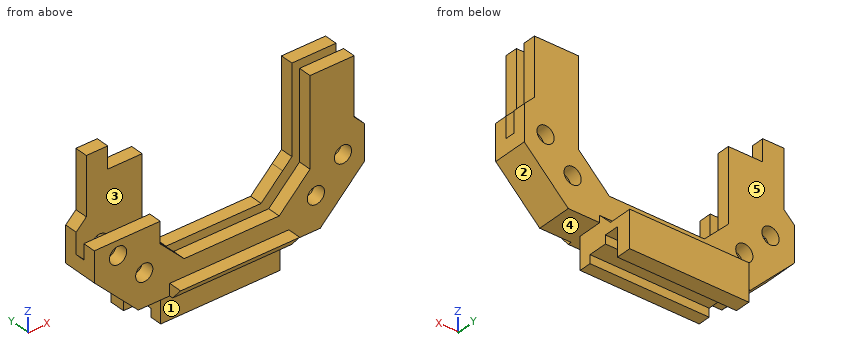
Autodesk Inventor part; units mm, degrees
ref_plane "Work Plane1" through (59.9208, 47.0911, 21.911) normal (0, 1, 0) x (-1, 0, 0)
ref_plane "Work Plane2" through (59.9208, 45.8611, 21.911) normal (0, -1, 0) x (1, 0, 0)
ref_plane "Work Plane13" through (59.9208, 43.8611, -18.7491) normal (1, 0, 0) x (0, 0, -1)
ref_plane "Work Plane1" through (59.9208, 47.0911, 21.911) normal (0, 1, 0) x (-1, 0, 0)
sketch "Sketch1" plane through (59.9208, 47.0911, 21.911) normal (0, 1, 0) x (-1, 0, 0)
  circle A0 centre (-16.808, -43.6345) radius 1.27
  circle A1 centre (12.5729, -47.6345) radius 1.27
  circle A2 centre (16.4459, -43.6345) radius 1.27
  circle A3 centre (-12.808, -47.6345) radius 1.27
  line L0 (10.208, -33.8805) -> (10.208, -44.6601)
  line L1 (10.208, -44.6601) -> (6.6725, -48.1956)
  circle A4 centre (-16.808, -43.6345) radius 1.27
  circle A5 centre (12.5729, -47.6345) radius 1.27
  circle A6 centre (16.4459, -43.6345) radius 1.27
  circle A7 centre (-12.8081, -47.6345) radius 1.27
  line L2 (19.708, -15.6655) -> (-19.708, -15.6655)
  line L3 (0, -15.6655) -> (0, -20.8781)
  line L4 (6.6725, -48.1956) -> (-7.3796, -48.1956)
  line L5 (-19.958, -43.8381) -> (-12.8316, -50.9645)
  line L6 (-12.8316, -50.9645) -> (12.8316, -50.9645)
  line L7 (-19.958, -40.6601) -> (-19.958, -43.8381)
  line L8 (0, -48.1956) -> (0, -46.7038)
  line L9 (19.958, -43.8381) -> (12.8316, -50.9645)
  line L10 (19.958, -40.6601) -> (19.958, -43.8381)
  line L11 (-11.938, -30.6601) -> (-11.938, -43.6372)
  line L12 (-10.5616, -45.0137) -> (-11.938, -43.6372)
  line L13 (-10.5616, -45.0137) -> (-7.3796, -48.1956)
  line L14 (15.2967, -30.6601) -> (18.458, -30.6601)
  line L15 (18.458, -30.6601) -> (18.458, -39.1601)
  line L16 (-18.458, -39.1601) -> (-18.458, -30.6601)
  line L17 (-18.458, -30.6601) -> (-11.938, -30.6601)
  line L18 (10.208, -33.8805) -> (15.2967, -33.8805)
  line L19 (15.2967, -33.8805) -> (15.2967, -30.6601)
  line L20 (-19.958, -40.6601) -> (-18.458, -39.1601)
  line L21 (19.958, -40.6601) -> (18.458, -39.1601)
  point P0 (-19.708, -43.6601)
  point P1 (-6.6725, -48.1956)
  dimension "d14" = 5
  dimension "d15" = 135
  dimension "d18" = 2.54
extrude "Extrusion1" add sketch "Sketch1" along normal blind 2
ref_plane "Work Plane2" through (59.9208, 45.8611, 21.911) normal (0, -1, 0) x (1, 0, 0)
sketch "Sketch2" plane through (59.9208, 45.8611, 21.911) normal (0, -1, 0) x (1, 0, 0)
  line L0 (-10.208, -33.8805) -> (-10.208, -44.6601)
  line L1 (-10.208, -44.6601) -> (-6.6725, -48.1956)
  line L2 (-6.6725, -48.1956) -> (7.3796, -48.1956)
  circle A0 centre (16.808, -43.6345) radius 1.27
  circle A1 centre (-12.5729, -47.6345) radius 1.27
  circle A2 centre (-16.4459, -43.6345) radius 1.27
  circle A3 centre (12.808, -47.6345) radius 1.27
  line L3 (19.958, -40.6601) -> (19.958, -43.8381)
  line L4 (19.958, -43.8381) -> (12.8316, -50.9645)
  line L5 (12.8316, -50.9645) -> (-12.8316, -50.9645)
  line L6 (-12.8316, -50.9645) -> (-19.958, -43.8381)
  line L7 (-19.958, -43.8381) -> (-19.958, -40.6601)
  line L8 (7.3796, -48.1956) -> (11.938, -43.6372)
  line L9 (11.938, -43.6372) -> (11.938, -30.6601)
  line L10 (11.938, -30.6601) -> (18.458, -30.6601)
  line L11 (18.458, -30.6601) -> (18.458, -39.1601)
  line L12 (-18.458, -39.1601) -> (-18.458, -30.6601)
  line L13 (-18.458, -30.6601) -> (-15.2967, -30.6601)
  line L14 (-15.2967, -30.6601) -> (-15.2967, -33.8805)
  line L15 (-15.2967, -33.8805) -> (-10.208, -33.8805)
  line L16 (18.458, -39.1601) -> (19.958, -40.6601)
  line L17 (-19.958, -40.6601) -> (-18.458, -39.1601)
  circle A4 centre (-16.4459, -43.6345) radius 1.27
  line L18 (-19.958, -43.8381) -> (-19.958, -40.6601)
  line L19 (-19.958, -41.5123) -> (-10.208, -41.5123)
  line L20 (-10.208, -33.8805) -> (-10.208, -44.6601)
  point P0 (-59.9208, -21.911)
extrude "Extrusion2" add sketch "Sketch2" along normal blind 2 contours L0 L1 L2 L8 L9 L10 L11 L16 L3 L4 L5 L6 L7 L19
sketch "Sketch4" plane through (79.8789, 45.8611, -18.7491) normal (1, 0, 0) x (0, 0, -1)
  line L0 (0, 1.23) -> (3.178, 1.23)
  line L1 (0, 0) -> (-1.5, 0)
  line L2 (0, 1.23) -> (0, 0)
  line L3 (-12.1065, -0.085) -> (12.1065, -0.085)
  line L4 (12.1065, -0.085) -> (12.1065, 1.315)
  line L5 (12.1065, 1.315) -> (-12.1065, 1.315)
  line L6 (-12.1065, 1.315) -> (-12.1065, -0.085)
  line L7 (-12.1065, -0.085) -> (12.1065, 1.315) construction
  line L8 (12.1065, -0.085) -> (-12.1065, 1.315) construction
  point P0 (0, 0.615)
  dimension "d73" = 1.4
extrude "Extrusion3" cut sketch "Sketch4" against normal through all
sketch "Sketch5" plane through (59.9208, 43.8611, 21.911) normal (0, -1, 0) x (1, 0, 0)
  line L0 (-19.708, -43.6601) -> (-19.708, -40.6601)
  line L1 (-12.6424, -50.7145) -> (-19.708, -43.6601)
  line L2 (12.728, -50.7145) -> (-12.6424, -50.7145)
  line L3 (19.708, -43.7345) -> (12.728, -50.7145)
  line L4 (-13.4529, -52.4645) -> (13.4529, -52.4645)
  line L5 (19.708, -43.7345) -> (19.708, -40.6601)
  line L6 (-12.8316, -50.9145) -> (12.8316, -50.9145)
  line L7 (12.8316, -50.9645) -> (11.3316, -52.4645)
  line L8 (-19.958, -43.8381) -> (-12.8316, -50.9645)
  line L9 (-12.8316, -50.9645) -> (-11.3316, -52.4645)
  line L10 (-12.8316, -50.9645) -> (-10.7103, -50.9645) construction
  line L11 (12.8316, -50.9145) -> (12.8816, -50.9145)
  line L12 (-12.8316, -50.9645) -> (12.8316, -50.9645)
  line L13 (12.8316, -50.9645) -> (12.8816, -50.9145)
  line L14 (12.8316, -50.9645) -> (19.958, -43.8381)
  line L15 (-12.8316, -50.9145) -> (-12.8816, -50.9145)
  line L16 (-12.8316, -50.9645) -> (-12.8816, -50.9145)
  line L17 (12.8109, -50.9145) -> (19.958, -43.7673)
  line L18 (-19.958, -43.7673) -> (-12.8109, -50.9145)
  line L19 (-19.958, -45.9594) -> (-13.4529, -52.4645)
  line L20 (13.4529, -52.4645) -> (19.958, -45.9594)
  line L21 (-19.958, -43.7673) -> (-19.958, -45.9594)
  line L22 (12.8316, -50.9645) -> (19.958, -43.8381)
  line L23 (19.958, -43.8381) -> (19.958, -45.9594)
  line L24 (19.958, -43.8381) -> (19.958, -43.7673)
  line L25 (19.958, -43.8381) -> (19.958, -40.6601)
  dimension "d29" = 0.2
  dimension "d62" = 45
  dimension "d74" = 0.05
  dimension "d75" = 0.05
  dimension "d76" = 1.5
  dimension "d77" = 1.5
extrude "Extrusion4" add sketch "Sketch5" against normal up to surface (5.23 mm away)
ref_plane "Work Plane13" through (59.9208, 43.8611, -18.7491) normal (1, 0, 0) x (0, 0, -1)
ref_plane "Work Plane14" through (53.2483, 46.4761, -26.2847) normal (0, 1, 0) x (1, 0, 0)
sketch "Sketch18" plane through (59.9208, 43.8611, -18.7491) normal (1, 0, 0) x (0, 0, -1)
  line L0 (12.8044, 1.651) -> (16.5534, 1.651)
  line L1 (16.5534, 1.651) -> (16.5534, 3.4515)
  line L2 (16.5534, 3.4515) -> (15.3033, 3.4515)
  line L3 (15.3033, 3.4515) -> (15.3033, 6.2794)
  line L4 (15.3033, 6.2794) -> (14.0544, 6.2794)
  line L5 (14.0544, 6.2794) -> (14.0544, 8.48)
  line L6 (14.0544, 8.48) -> (18.2804, 8.48)
  line L7 (18.2804, 8.48) -> (18.2804, 10.73)
  line L8 (18.2804, 10.73) -> (12.8044, 10.73)
  line L9 (12.8044, 7.23) -> (12.8044, 10.73)
  line L10 (11.8044, 0) -> (11.8044, 5.23)
  line L11 (11.8044, 5.23) -> (11.8044, 0)
  line L12 (11.8044, 5.23) -> (10.8044, 5.23)
  line L13 (12.8044, 1.651) -> (11.8044, 1.651)
  line L14 (12.8044, 7.23) -> (10.8044, 5.23)
  line L15 (11.8044, 0) -> (10.0544, 0)
  line L16 (10.0544, 0) -> (10.0544, -2)
  line L17 (10.0544, -2) -> (11.8044, -0.5316)
  line L18 (11.8044, -0.5316) -> (11.8044, 0)
  point P0 (12.8044, 5.23)
  point P1 (11.8044, 1.651)
  dimension "d182" = 2
  dimension "d183" = 2
  dimension "d184" = 1.75
  dimension "d185" = 2
  dimension "d186" = 50
extrude "Extrusion12" add sketch "Sketch18" along normal blind 8.804 and the other way blind 8.804
ref_plane "Work Plane19" through (51.1168, 52.1911, -37.0296) normal (0, -1, 0) x (1, 0, 0)
ref_plane "Work Plane20" through (68.7248, 50.1406, -34.2524) normal (0, 0, -1) x (-1, 0, 0)
properties part number "Button Holder"
Here's how the part is built. I have some questions about the finished solid (model axes, mm). Face numbers are marked on the shaded views. A direction names the side the tool comes from. Give positions to 0.01 mm unless a question says otherwise; leave off trailing zeros. Order: outer loops, then holes, each group sorted by start corner. A loop starts at its lowest first (then second) coordinate and runs counter-clockwise, first axis right, second up. Notation, with made-up numbers: (55, 74.5) - (69, 74.5) arc R15 cw to (69, 96.5) - close; hole circle Ø11 at (80.25, 52). An arc over 180 degrees is marked (long way). Answer as a JSON object with one key per item and string values. Group by question number.
Item 1: If we mould it in two halves opening along Y, with no side actions, what happens to the marked faces 3, 4 and 5? For each: pulls with the +Y half, pulls with the -Y half, needs draft (parallel to the pull), parting line crosses it, or undercut.
Item 2: If we section it at B-B on x = 55: Please give me the cut outline in (y, z), and give its area (3 significant figures).
Item 3: If we section it at D-D on z = -16.5: Please give me the cut outline in (x, y).
Item 4: If we section it at C-C on y = 47.75: Please give me the cut outline in (x, z), and give its area (3 significant figures).
Item 5: Please list where these lines run through material, in increasing order: probe 1 along X at (y, z) = (47.25, -15.25); probe 2 along Y at (x, z) = (76, -19.25); probe 3 along Z at (x, y) = (59.5, 52.75).
Item 6: For P1, Ø5, axis at x = 57, z = -24, coming from the +Y side; P2, Ø8, axis at x = 65, z = -15, coming from the -Y side; P3, Ø1.6, axis at x = 59.5, y = 43, coming from the +Z side; P4, Ø1, axis at y = 48, z = -12.5, coming from the -X side, each with a flat end and sliding along its axis, tell me the tip position at first contact or that it passes through.
Item 7: Which directions (+Z, -Z, +X, -X, +Y, -Y) give clear straight access to the entire face, cutting with the end or side of a thin tool? Please do the marked faces 1 and 2.
Item 8: If we section it at A-A on z = -10.75: Please give me the cut outline in (x, y).
Result set:
{
 "1": {"face 3": "undercut", "face 4": "needs draft", "face 5": "pulls with the +Y half"},
 "2": {"outline": "(41.86, -28.8) - (43.33, -30.55) - (45.51, -30.55) - (45.51, -35.3) - (47.31, -35.3) - (47.31, -34.05) - (50.14, -34.05) - (50.14, -32.8) - (52.34, -32.8) - (52.34, -37.03) - (54.59, -37.03) - (54.59, -31.55) - (51.09, -31.55) - (49.09, -29.55) - (49.09, -26.28) - (47.18, -26.28) - (47.18, -29) - (45.78, -29) - (45.78, -26.28) - (43.86, -26.28) - (43.86, -28.8) - close", "area": "55.2 mm²"},
 "3": {"outline": "(41.46, 47.18) - (49.71, 47.18) - (49.71, 49.09) - (41.46, 49.09) - close; (71.86, 43.86) - (78.38, 43.86) - (78.38, 45.78) - (71.86, 45.78) - close; (71.86, 47.18) - (78.38, 47.18) - (78.38, 49.09) - (71.86, 49.09) - close"},
 "4": {"outline": "(39.96, -24.05) - (46.47, -30.55) - (51.12, -30.55) - (51.12, -34.05) - (68.72, -34.05) - (68.72, -30.55) - (73.37, -30.55) - (79.88, -24.05) - (79.88, -18.75) - (78.38, -17.25) - (78.38, -8.75) - (71.86, -8.75) - (71.86, -21.73) - (70.48, -23.1) - (67.3, -26.28) - (53.25, -26.28) - (49.71, -22.75) - (49.71, -11.97) - (44.62, -11.97) - (44.62, -8.75) - (41.46, -8.75) - (41.46, -17.25) - (39.96, -18.75) - close; hole circle Ø2.54 at (43.47, -21.72); hole circle Ø2.54 at (47.35, -25.72); hole circle Ø2.54 at (72.73, -25.72); hole circle Ø2.54 at (76.73, -21.72)", "area": "454 mm²"},
 "5": {"probe 1": "41.46 to 49.71, 71.86 to 78.38", "probe 2": "43.86 to 45.78, 47.18 to 49.09", "probe 3": "-37.03 to -31.55"},
 "6": {"P1": "y = 49.09", "P2": "through", "P3": "z = -28.8", "P4": "x = 41.46"},
 "7": {"face 1": "-Z, +X, -X, -Y", "face 2": "-Z, +X, +Y, -Y"},
 "8": {"outline": "(41.46, 47.18) - (44.62, 47.18) - (44.62, 49.09) - (41.46, 49.09) - close; (71.86, 43.86) - (78.38, 43.86) - (78.38, 45.78) - (71.86, 45.78) - close; (71.86, 47.18) - (78.38, 47.18) - (78.38, 49.09) - (71.86, 49.09) - close"}
}
